Verification items for the finished model (mm, model axes). Give positions to 0.01 mm unless a question says otherwise; leave off trailing zeros. Order: outer loops, then holes, each group sorted by start corner. A loop starts at its lowest first (then second) coordinate and runs counter-clockwise, first axis right, second up.
Autodesk Inventor part; units mm, degrees
ref_plane "YZ Plane" through (0, 0, 0) normal (1, 0, 0) x (0, 1, 0)
ref_plane "XZ Plane" through (0, 0, 0) normal (0, 1, 0) x (-1, 0, 0)
ref_plane "XY Plane" through (0, 0, 0) normal (0, 0, 1) x (1, 0, 0)
sketch "スケッチ1" plane through (0, 0, 0) normal (0, 1, 0) x (-1, 0, 0)
  line L0 (0, 99) -> (30, 99)
  line L1 (30, 99) -> (30, -99)
  line L2 (30, -99) -> (0, -99)
  line L3 (0, -99) -> (0, 99)
  line L4 (0, -69) -> (15, -69)
  line L5 (15, -69) -> (15, 0)
  line L6 (36, 0) -> (-6, 0)
  line L7 (0, 69) -> (15, 69)
  line L8 (15, 69) -> (15, 0)
  point P0 (0, 0)
  point P1 (0, 0)
  dimension "d0" = 198
  dimension "d1" = 30
  dimension "d32" = 30
  dimension "d33" = 15
extrude "押し出し1" add sketch "スケッチ1" along normal blind 2.5 contours L0 L1 L6 L8 L7 L3 | L1 L2 L3 L4 L5 L6
properties part number "belt_rail" material "木材 (カエデ材)"
(1) Section check A-A, the plane x = -9.5. Enter the section's corners in (y, z), then the cut area to 3 significant figures.
Solved:
outline: (0, -99) - (2.5, -99) - (2.5, -69) - (0, -69) - close; (0, 69) - (2.5, 69) - (2.5, 99) - (0, 99) - close
area: 150 mm2
(2) Go/stop test with a flat-tipped pin: pin 1 (1 mm diameter, centred on y = 0.5, z = -23.5, fed in from +X). Record where the tip stops, or that it passes through.
Solved:
pin 1: stops at x = -15
(3) Section check B-B, the plane y = 0.7. Enter the section's corners in (x, z), then the cut area to 3 significant figures.
Solved:
outline: (-30, -99) - (0, -99) - (0, -69) - (-15, -69) - (-15, 69) - (0, 69) - (0, 99) - (-30, 99) - close
area: 3,870 mm2
(4) Scan lines: line 1 (Z direction, x = -4.5, y = 1.1); line 2 (X direction, y = 0.8, z = 23). Record each from-to range of solid material in increasing order.
Solved:
line 1: z = -99 to -69, 69 to 99
line 2: x = -30 to -15
(5) Section check C-C, the plane z = 65. Enter the section's corners in (x, y).
Solved:
outline: (-30, 0) - (-15, 0) - (-15, 2.5) - (-30, 2.5) - close
